```python
from build123d import *

# Parameters (mm, degrees)
F1_DEPTH = 88.9
F2_DEPTH = 38.1


with BuildPart() as f1:
    # F0 (on Front) → F1 (new body)
    with BuildSketch(Plane.XZ):
        Polygon((101.6, 340.150816), (-101.6, 543.350816), (-101.6, -552.244648), (101.6, -349.044648), align=None)
        Polygon((101.6, -349.044648), (-101.6, -552.244648), (-74.659232, -579.185416), (101.6, -402.926184), align=None)
        Polygon((-74.659232, 570.291584), (-101.6, 543.350816), (101.6, 340.150816), (101.6, 394.032352), align=None)
    extrude(amount=F1_DEPTH)

    # F0 (on Front) → F2 (join)
    with BuildSketch(Plane.XZ):
        Polygon((101.6, 394.032352), (101.6, 519.755938), (-11.797439, 633.153377), (-74.659232, 570.291584), align=None)
        Polygon((101.6, -402.926184), (-74.659232, -579.185416), (-11.797439, -642.047209), (101.6, -528.64977), align=None)
    extrude(amount=F2_DEPTH)


solid = f1.part
```
Model file for the job. Use its own axes, mm. A direction names the side the tool comes from. Coordinates: 2 decimals unless noted, no trailing zeros. Order: outer loops, then holes, each group sorted by start corner. A loop starts at its lowest first (then second) coordinate and runs counter-clockwise, first axis right, second up. Notation, with made-up numbers: (17, 56) -> (51, 56) arc R28 ccw to (51, 93) -> close; hole circle Ø11 at (-11, 40). An arc over 180 degrees is marked (long way). Return JSON: item names as keys, results as strings.
Item 1: Slice it at A-A (y = -69.5). Write the cut outline in (x, z), then the cut area to 3 significant figures.
Model answer:
{"outline": "(-101.6, -552.24) -> (-74.66, -579.19) -> (101.6, -402.93) -> (101.6, 394.03) -> (-74.66, 570.29) -> (-101.6, 543.35) -> close", "area": "202,000 mm²"}
Item 2: Slice it at C-C (z = -480). Write the cut outline in (x, y).
Model answer:
{"outline": "(-101.6, -88.9) -> (24.53, -88.9) -> (24.53, -38.1) -> (101.6, -38.1) -> (101.6, 0) -> (-101.6, 0) -> close"}
Item 3: Pin check, flat tips, straight feed: P1, Ø2, axis at x = 10, y = -50.5, coming from the +Z side; P2, Ø3, axis at y = -78.5, z = -454.5, coming from the +X side; P3, Ø2, axis at x = -6.5, y = -21, coming from the +Z side. Stop position of each tip, or through.
Model answer:
{"P1": "stops at z = 486.63", "P2": "stops at x = 51.53", "P3": "stops at z = 628.86"}
Item 4: 3-axis set-ups, long thin cutter, end or side, ignore diameter. For faces 1 (the face through (12.237, -63.144, -492.29)), 2 (the face through (32, -38.1, 515)), 3 (the face through (45.695, -18.783, 575.661)): which of +Z, -Z, +X, -X, +Y, -Y reach the whole face in a straight line?
Model answer:
{"face 1": "-Z, +X, -Y", "face 2": "+Z, +X, -Y", "face 3": "+Z, +X, +Y, -Y"}
Item 5: Slice it at D-D (x = 84). Write the cut outline in (y, z), then the cut area to 3 significant figures.
Model answer:
{"outline": "(-88.9, -420.53) -> (-38.1, -420.53) -> (-38.1, -546.25) -> (0, -546.25) -> (0, 537.36) -> (-38.1, 537.36) -> (-38.1, 411.63) -> (-88.9, 411.63) -> close", "area": "83,600 mm²"}
Item 6: Slice it at B-B (x = -25). Write the cut outline in (y, z).
Model answer:
{"outline": "(-88.9, -529.53) -> (-38.1, -529.53) -> (-38.1, -628.84) -> (0, -628.84) -> (0, 619.95) -> (-38.1, 619.95) -> (-38.1, 520.63) -> (-88.9, 520.63) -> close"}
Item 7: Wall check: line 1 along Y through (x, z) = (-7.5, -588); line 2 along Z through (x, y) = (-14, -50.5); line 3 along Z through (x, y) = (12, -62). Give the ranges that are in metal, low to high. Write a range as from..to.
Model answer:
{"line 1": "y = -38.1..0", "line 2": "z = -518.53..509.63", "line 3": "z = -492.53..483.63"}
